The drawing under review shows one solid part. Ordinate dimensions are in mm from its lowest x, y, z. A direction names the side the tool comes from. Give positions to 0.01 mm unless a question says otherwise; leave off trailing zeros. Loops run counter-clockwise (first coordinate to the right, second up) from the corner with the lowest first, then second, coordinate; pieces in that order, holes last. Notation, with made-up numbers: M 27,-35.5 L 34,-35.5 A15 ccw 34,-14.5 Z; hole C 20.25,-11 d9. An arc over 180 degrees is marked long. Write item = value, one per line. Start each with the question number.
1. For pin 1 (1.5 mm diameter, centred on x = 5.5, z = 17, fed in from -Y); pin 2 (6 mm diameter, centred on x = 12.5, y = 35.5, fed in from +Z); pin 3 (6.5 mm diameter, centred on y = 8.44, z = 15.07, fed in from -X), all flat-tipped, find the tip position at first contact; note any pin that passes through.
2. Wall thickness on line 1 along X through (y, z) = (34, 13.25); line 2 along Y through (x, z) = (14, 11.25): over which ranges is each line inside the solid? List them lowest first. Write a range as from..to.
3. We need section A-A on y = 34. Give the boundary of the cut face in (x, z), then the cut area to 3 significant figures.
4. For the marked faces 1 and 2, list the 3-axis set-ups (+Z, -Z, +X, -X, +Y, -Y) from which the entire face can be reached by the end or side of a thin tool; tool diameter is ignored.
5. We need section B-B on z = 4. Give the boundary of the cut face in (x, y).
6. We need section D-D on x = 10. Give the boundary of the cut face in (y, z).
7. Draft analysis for pull direction X (two halves, no side actions). For the marked faces 3, 4 and 5, state which applies: pulls with the +X half, pulls with the -X half, needs draft (parallel to the pull), parting line crosses it, or undercut.
8. We need section C-C on z = 16. Count the separate pieces of the cut face and the enclosed holes in it, then the cut area to 3 significant figures.
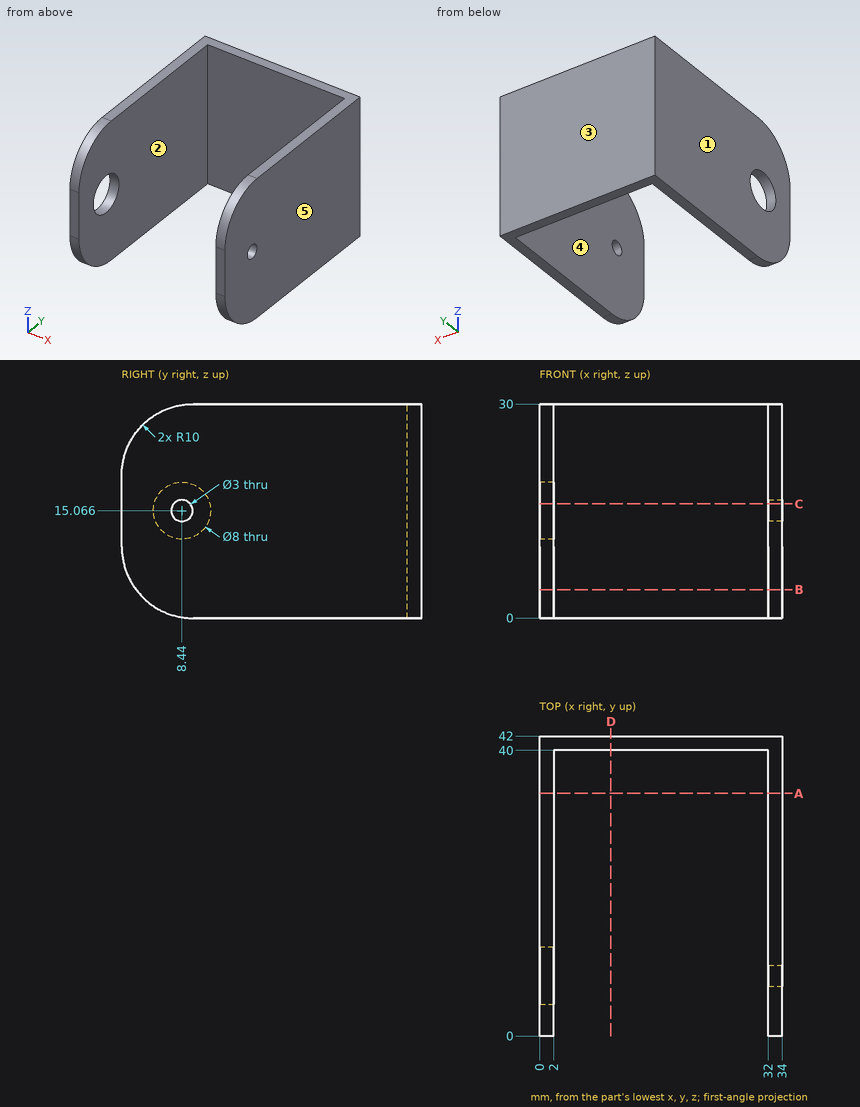
Final values:
q1.pin_1 = 40
q1.pin_2 = through
q1.pin_3 = 32
q2.line_1 = 0..2, 32..34
q2.line_2 = 40..42
q3.outline = M 0,0 L 2,0 L 2,30 L 0,30 Z; M 32,0 L 34,0 L 34,30 L 32,30 Z
q3.area = 120 mm²
q4.face_1 = +Z, -Z, -X, +Y, -Y
q4.face_2 = +Z, -Z, -Y
q5.outline = M 0,2 L 2,2 L 2,40 L 32,40 L 32,2 L 34,2 L 34,42 L 0,42 Z
q6.outline = M 40,0 L 42,0 L 42,30 L 40,30 Z
q7.face_3 = needs draft
q7.face_4 = undercut
q7.face_5 = pulls with the +X half
q8.separate_pieces = 3
q8.enclosed_holes = 0
q8.area = 208 mm²
